from build123d import *

# Parameters (mm, degrees)
F0_R     = 25.4
F1_DEPTH = 12.7
F3_DEPTH = 12.7
F5_COUNT = 6
F6_R     = 6.35
F7_DEPTH = 25.4
F8_T     = -2.54


with BuildPart() as f1:
    # F0 (on Top) → F1 (new body)
    with BuildSketch(Plane.XY):
        Circle(F0_R)
    extrude(amount=F1_DEPTH)

    # F2 (on face) → F3 (join)
    with BuildSketch(Plane.XY.offset(12.7)):
        Polygon((-6.5740037456, 24.5345159877), (0, 0), (0, 24.5345159877), align=None)
        Polygon((0, 24.5345159877), (0, 0), (6.5740037456, 24.5345159877), align=None)
        Polygon((-6.5740037456, 24.5345159877), (0, 24.5345159877), (6.5740037456, 24.5345159877), (6.5740037456, 34.6945151687), (-6.5740037456, 34.6945151687), align=None)
    extrude(amount=-F3_DEPTH)

    # F5: F1 ×6 about axis
    f5_axis = Axis((0, 0, 27.9026478529), (0, 0, 1))


with BuildPart() as f1_1:
    add(f1.part)
    for i in range(1, F5_COUNT):
        add(f1.part.rotate(f5_axis, i * 360 / F5_COUNT))

    # F6 (on face) → F7 (cut)
    with BuildSketch(Plane.XY.offset(12.7)):
        Circle(F6_R)
    extrude(amount=-F7_DEPTH, mode=Mode.SUBTRACT)

    # F8
    f8_openings = [f1_1.faces().sort_by_distance(p)[0] for p in [
        (-24.437748, 0, 0),
    ]]
    offset(amount=F8_T, openings=f8_openings, kind=Kind.INTERSECTION)


solid = f1_1.part
Design review of the part built by this model. Coordinates are the model's own, in mm. A direction names the side the tool comes from. Coordinates: 2 decimals unless noted, no trailing zeros. Order: outer loops, then holes, each group sorted by start corner. A loop starts at its lowest first (then second) coordinate and runs counter-clockwise, first axis right, second up. Notation, with made-up numbers: (87.25, 56) - (100.25, 56) arc R19 ccw to (100.25, 81) - close; hole circle Ø1 at (84, 71.5). An arc over 180 degrees is marked (long way). Put each result on its own line as item: value.
1) Take a section at B-B, the plane z = 11. Give the boundary of the cut face in (x, y), and give its area (3 significant figures).
Response values:
outline: (-33.33, -11.65) - (-26.76, -23.04) - (-17.96, -17.96) arc R25.4 ccw to (-6.57, -24.53) - (-6.57, -34.69) - (6.57, -34.69) - (6.57, -24.53) arc R25.4 ccw to (17.96, -17.96) - (26.76, -23.04) - (33.33, -11.65) - (24.53, -6.57) arc R25.4 ccw to (24.53, 6.57) - (33.33, 11.65) - (26.76, 23.04) - (17.96, 17.96) arc R25.4 ccw to (6.57, 24.53) - (6.57, 34.69) - (-6.57, 34.69) - (-6.57, 24.53) arc R25.4 ccw to (-17.96, 17.96) - (-26.76, 23.04) - (-33.33, 11.65) - (-24.53, 6.57) arc R25.4 ccw to (-24.53, -6.57) - close; hole circle Ø12.7 at (0, 0)
area: 2,660 mm²
2) Insertion check: P1, Ø3, axis at x = 25, z = 11, coming from the -Y side; P2, Ø1.5, axis at x = -14.5, z = 3.5, coming from the +Y side; P3, Ø1.5, axis at y = 18, z = 2.5, coming from the -X side. Each pin has a flat end and moves straight along its axis. Give the tip position at first contact, or say it passes through.
Response values:
P1: stops at y = -22.89
P2: stops at y = 21.36
P3: stops at x = -30.1
3) Wall thickness on L1, parallel to Y at x = 0, z = 4.75; L2, parallel to X at y = 30.5, z = 8.25; L3, parallel to X at y = 4, z = 8.5: over which ranges is each line inside the solid? List them lowest first. Write a range as from..to.
Response values:
L1: y = -34.69..-32.15, -8.89..-6.35, 6.35..8.89, 32.15..34.69
L2: x = -6.57..-4.03, 4.03..6.57
L3: x = -25.08..-22.51, -7.94..-4.93, 4.93..7.94, 22.51..25.08
4) Take a section at C-C, the plane x = 0. Give the boundary of the cut face in (y, z), and give its area (3 significant figures).
Response values:
outline: (-34.69, 0) - (-32.15, 0) - (-32.15, 10.16) - (-8.89, 10.16) - (-8.89, 0) - (-6.35, 0) - (-6.35, 12.7) - (-34.69, 12.7) - close; (6.35, 0) - (8.89, 0) - (8.89, 10.16) - (32.15, 10.16) - (32.15, 0) - (34.69, 0) - (34.69, 12.7) - (6.35, 12.7) - close
area: 247 mm²
5) The part is to be moulded in two halves that separate along Y. For faces 4 (the face through (-30, 17.43, 6.44)), 5 (the face through (6.574, 30, 6)), 6 (the face through (21.708, 17.191, 5.151)), say which applies: released by +Y, released by -Y, zero draft, split by the parting line, or undercut.
Response values:
face 4: released by +Y
face 5: zero draft
face 6: undercut
6) Take a section at D-D, the plane y = -26.5. Give the boundary of the cut face in (x, z), and give its area (3 significant figures).
Response values:
outline: (-6.57, 0) - (-4.03, 0) - (-4.03, 10.16) - (4.03, 10.16) - (4.03, 0) - (6.57, 0) - (6.57, 12.7) - (-6.57, 12.7) - close
area: 85.0 mm²
7) Take a section at A-A, the plane y = 0. Give the boundary of the cut face in (x, z).
Response values:
outline: (-25.4, 0) - (-22.86, 0) - (-22.86, 10.16) - (-8.89, 10.16) - (-8.89, 0) - (-6.35, 0) - (-6.35, 12.7) - (-25.4, 12.7) - close; (6.35, 0) - (8.89, 0) - (8.89, 10.16) - (22.86, 10.16) - (22.86, 0) - (25.4, 0) - (25.4, 12.7) - (6.35, 12.7) - close
8) Tool access review of faces 1 (the face through (-29, 9.15, 6.44)), 2 (the face through (-3, -9, 10.16)), 3 (the face through (-6.574, 30, 6)): name each direction out of +Z, -Z, +X, -X, +Y, -Y from which nothing blocks a thin tool from reaching the whole face with its end or side.
Response values:
face 1: +Z, -Z, -X
face 2: -Z
face 3: +Z, -Z, -X, +Y
